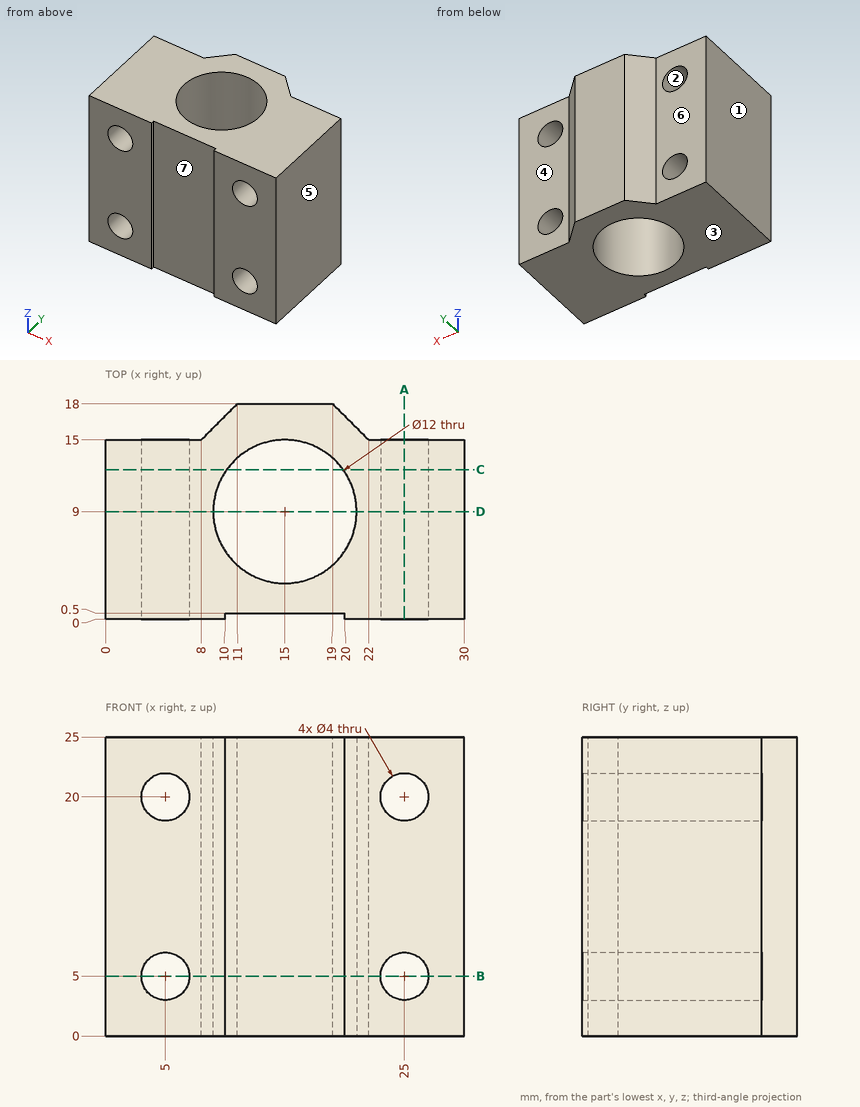
Could you check a few things on this drawing? It's one solid part, dimensions in mm from its lowest x, y, z. A direction names the side the tool comes from. Give positions to 0.01 mm unless a question says otherwise; leave off trailing zeros. Loops run counter-clockwise (first coordinate to the right, second up) from the corner with the lowest first, then second, coordinate; pieces in that order, holes last. Notation, with made-up numbers: M 77,-12 L 116,-12 A27 ccw 116,25 Z; hole C -22,60 d10. An arc over 180 degrees is marked long. Answer as a JSON object with one key per item and string values.
Q1. If I drill on probe 1 along Z at (x, y) = (25, 5); probe 2 along X at (y, z) = (3.75, 4); probe 3 along Z at (x, y) = (23.25, 7.75), over which ranges is the centre line in solid material (lowest first)? Write a range as [from, to].
Values found:
{"probe 1": "z = [0, 3], [7, 18], [22, 25]", "probe 2": "x = [0, 3.27], [6.73, 12.1], [17.9, 23.27], [26.73, 30]", "probe 3": "z = [0, 4.03], [5.97, 19.03], [20.97, 25]"}
Q2. Suppose I cut it at A-A, the plane x = 25. List the corners of the cut face in (y, z) for me.
Values found:
{"outline": "M 0,0 L 15,0 L 15,3 L 0,3 Z; M 0,7 L 15,7 L 15,18 L 0,18 Z; M 0,22 L 15,22 L 15,25 L 0,25 Z"}
Q3. Suppose I cut it at C-C, the plane y = 12.5. List the corners of the cut face in (x, z) for me.
Values found:
{"outline": "M 0,0 L 10.13,0 L 10.13,25 L 0,25 Z; M 19.87,0 L 30,0 L 30,25 L 19.87,25 Z; hole C 5,5 d4; hole C 5,20 d4; hole C 25,5 d4; hole C 25,20 d4"}
Q4. Suppose I cut it at D-D, the plane y = 9. List the corners of the cut face in (x, z) for me.
Values found:
{"outline": "M 0,0 L 9,0 L 9,25 L 0,25 Z; M 21,0 L 30,0 L 30,25 L 21,25 Z; hole C 5,5 d4; hole C 5,20 d4; hole C 25,5 d4; hole C 25,20 d4"}
Q5. For P1, Ø2.5, axis at x = 26, z = 15, coming from the +Y side; P2, Ø5, axis at x = 23, z = 5.5, coming from the +Y side; P3, Ø3, axis at x = 14.5, z = 6.5, coming from the -Y side, each with a flat end and sliding along its axis, tell me the tip position at first contact or that it passes through.
Values found:
{"P1": "stops at y = 15", "P2": "stops at y = 16.5", "P3": "stops at y = 0.5"}
Q6. If we mould it in two halves opening along Z, with no side actions, what happens to the marked faces 1, 2 and 3? For each: pulls with the +Z half, pulls with the -Z half, needs draft (parallel to the pull), parting line crosses it, or undercut.
Values found:
{"face 1": "needs draft", "face 2": "undercut", "face 3": "pulls with the -Z half"}
Q7. For the marked faces 4, 5, 6 and 7, which set-ups out of +Z, -Z, +X, -X, +Y, -Y let a thin tool reach every point of the face, with its end or its side?
Values found:
{"face 4": "+Z, -Z, +X, +Y", "face 5": "+Z, -Z, +X, +Y, -Y", "face 6": "+Z, -Z, -X, +Y", "face 7": "+Z, -Z, -Y"}
Q8. Suppose I cut it at B-B, the plane z = 5. List the corners of the cut face in (x, y) for me, plus the area to 3 significant figures.
Values found:
{"outline": "M 0,0 L 3,0 L 3,15 L 0,15 Z; M 7,0 L 10,0 L 10,0.5 L 20,0.5 L 20,0 L 23,0 L 23,15 L 22,15 L 19,18 L 11,18 L 8,15 L 7,15 Z; M 27,0 L 30,0 L 30,15 L 27,15 Z; hole C 15,9 d12", "area": "245 mm²"}
